Can you work these out from the model? Positions are in its coordinate system, mm. Face numbers are marked on the shaded views. Coordinates: 2 decimals unless noted, no trailing zeros. Order: outer loops, then holes, each group sorted by start corner. A loop starts at its lowest first (then second) coordinate and runs counter-clockwise, first axis right, second up.
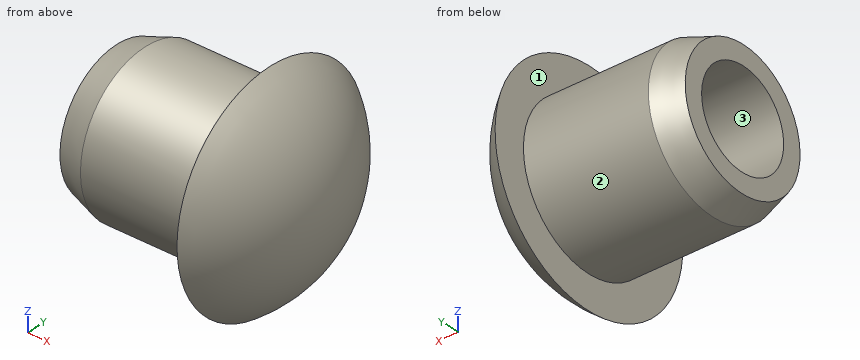
```python
from build123d import *


with BuildPart() as part:
    # 草图1 → 旋转1 (revolve)
    with BuildSketch(Plane.XY, mode=Mode.PRIVATE) as revolve_1_sk:
        with BuildLine():
            Line((0, 2.5), (0, 3.5))
            Line((0, 3.5), (1.494559039, 4))
            Line((1.494559039, 4), (8, 4))
            Line((8, 4), (8, 5.726362631))
            ThreePointArc((8, 5.726362631), (10.173497708, 3.222185879), (10.956128949, 0))
            Line((10.956128949, 0), (8, 0))
            Line((8, 0), (8, 2.5))
            Line((8, 2.5), (0, 2.5))
        make_face()
    revolve(revolve_1_sk.sketch.rotate(Axis((0, 0, 0), (1, 0, 0)), 90), axis=Axis((0, 0, 0), (1, 0, 0)))


solid = part.part
```
1. Thinking about a two-plate mould opening in Y: for the marked faces 1, 2 and 3, which applies, pulls with the +Y half, pulls with the -Y half, needs draft (parallel to the pull), parting line crosses it, or undercut?
Completed:
face 1: needs draft
face 2: parting line crosses it
face 3: undercut
2. Imagine slicing it at A-A on z = 0. Please give me the cut outline in (x, y), then the cut area to 3 significant figures.
Completed:
outline: (0, -3.5) - (1.49, -4) - (8, -4) - (8, -5.73) arc R7.02 ccw to (8, 5.73) - (8, 4) - (1.49, 4) - (0, 3.5) - (0, 2.5) - (8, 2.5) - (8, -2.5) - (0, -2.5) - close
area: 47.0 mm2
3. Imagine slicing it at C-C on x = 1.25. Please give me the cut outline in (y, z).
Completed:
outline: circle Ø7.84 at (0, 0); hole circle Ø5 at (0, 0)
4. Imagine slicing it at D-D on x = 2.75. Please give me the cut outline in (y, z), then the cut area to 3 significant figures.
Completed:
outline: circle Ø8 at (0, 0); hole circle Ø5 at (0, 0)
area: 30.6 mm2
5. Please list where these lines run through material, in increasing order: probe 1 along Y at (x, z) = (6.25, 0); probe 2 along Z at (x, y) = (7, 1.5); probe 3 along Z at (x, y) = (6.75, -2).
Completed:
probe 1: y = -4 to -2.5, 2.5 to 4
probe 2: z = -3.71 to -2, 2 to 3.71
probe 3: z = -3.46 to -1.5, 1.5 to 3.46
6. I'm going to push flat-ended pins straight in: pin 1 (3 mm diameter, centred on x = 2.5, z = 1, fed in from -Y); pin 2 (3 mm diameter, centred on x = 1.5, y = 3.5, fed in from +Z); pin 3 (3 mm diameter, centred on x = 5.5, y = 0, fed in from +Z). Where does each tip first touch, or does it pass through?
Completed:
pin 1: stops at y = -4
pin 2: stops at z = 3.46
pin 3: stops at z = 4
